Can you work these out from the model? Positions are in its coordinate system, mm. Face numbers are marked on the shaded views. A direction names the side the tool comes from. Coordinates: 2 decimals unless noted, no trailing zeros. Write each loop counter-clockwise with the first axis right and the second up, starting at its lowest first coordinate (ties: lowest second). Pieces come first, ordered by that corner, then holes. Notation, with made-up numbers: (25, 31) - (35, 31) arc R20 cw to (35, 51) - close; hole circle Ø6 at (25.25, 18.5). An arc over 180 degrees is marked (long way). Use one line per item in the form item = value. Start each with the question number.
(1) Thinking about a two-plate mould opening in X: for the marked faces 1, 2, 3 and 4, which applies, pulls with the +X half, pulls with the -X half, needs draft (parallel to the pull), parting line crosses it, or undercut?
(2) On a 3-axis mill with a long thin cutter (end or side, diameter ignored), from which of +Z, -Z, +X, -X, +Y, -Y can I reach the whole of each face in a straight line? I mean the marked faces 5, 6 and 7. Say none if no direction works.
(3) For pin 1 Ø2.5 at (x, y) = (-47.45, 55.69) entering from +Z; pin 2 Ø2 at (y, z) = (32.5, -28) entering from +X; pin 3 Ø17.5 at (y, z) = (37, -6) entering from +X; pin 4 Ø0.5 at (y, z) = (63.5, 3.5) entering from +X, each with a flat end and sliding along its axis, tell me the tip position at first contact or that it passes through.
(4) If we section it at A-A on z = -24.5: Please give me the cut outline in (x, y), then the cut area to 3 significant figures.
(5) If I drill on probe 1 along X at (y, z) = (-3, -12); probe 2 along X at (y, z) = (11.5, -16); probe 3 along Y at (x, z) = (54.5, -18), over which ranges is the centre line in solid material (lowest first)? Write a range as from..to.
Autodesk Fusion 360 part; units mm, degrees
sketch "Schizzo1" plane through (0, 0, 0) normal (0, 0, 1) x (1, 0, 0)
  line L0 (-31.0508, 65.6855) -> (44.1492, 65.6855)
  line L1 (44.1492, 65.6855) -> (44.1492, -9.3145)
  line L2 (44.1492, -9.3145) -> (-31.0508, -9.3145)
  line L3 (-31.0508, -9.3145) -> (-31.0508, 65.6855)
  line L4 (-31.0508, 28.1855) -> (44.1492, 28.1855) construction
  line L5 (6.5492, 65.6855) -> (6.5492, -9.3145) construction
  circle A0 centre (6.5492, 28.1855) radius 30.5
  line L6 (37.0492, -2.3145) -> (-23.9508, -2.3145) construction
  line L7 (-23.9508, -2.3145) -> (-23.9508, 58.6855) construction
  line L8 (-23.9508, 58.6855) -> (37.0492, 58.6855) construction
  line L9 (37.0492, 58.6855) -> (37.0492, -2.3145) construction
  line L10 (37.0492, -2.3145) -> (-23.9508, 58.6855) construction
  line L11 (-23.9508, -2.3145) -> (37.0492, 58.6855) construction
  circle A1 centre (-23.9508, 58.6855) radius 2.1
  circle A2 centre (37.0492, 58.6855) radius 2.1
  circle A3 centre (37.0492, -2.3145) radius 2.1
  circle A4 centre (-23.9508, -2.3145) radius 2.1
  line L12 (-71.9508, 58.6855) -> (-66.9508, 58.6855)
  line L13 (-66.9508, 58.6855) -> (-66.9508, -2.3145)
  line L14 (-66.9508, -2.3145) -> (-71.9508, -2.3145)
  line L15 (-71.9508, -2.3145) -> (-71.9508, 58.6855)
  line L16 (85.0492, 58.6855) -> (80.0492, 58.6855)
  line L17 (85.0492, -2.3145) -> (85.0492, 58.6855)
  line L18 (80.0492, 58.6855) -> (80.0492, -2.3145)
  line L19 (80.0492, -2.3145) -> (85.0492, -2.3145)
  circle A5 centre (-23.9508, 58.6855) radius 3.6
  circle A6 centre (37.0492, 58.6855) radius 3.6
  circle A7 centre (-23.9508, -2.3145) radius 3.6
  circle A8 centre (37.0492, -2.3145) radius 3.6
  line L20 (-31.0508, -9.3145) -> (-71.9508, -9.3145)
  line L21 (-71.9508, -9.3145) -> (-71.9508, -2.3145)
  line L22 (44.1492, -9.3145) -> (85.0492, -9.3145)
  line L23 (85.0492, -9.3145) -> (85.0492, -2.3145)
  line L24 (-66.9508, -2.3145) -> (-66.9508, -9.3145)
  line L25 (80.0492, -2.3145) -> (80.0492, -9.3145)
  line L26 (-66.9508, 58.6855) -> (-31.0508, 58.6855)
  line L27 (80.0492, 58.6855) -> (44.1492, 58.6855)
  line L28 (-66.9508, 58.6855) -> (-31.0508, 58.6855)
  line L29 (-31.0508, 58.6855) -> (-31.0508, 60.6855)
  line L30 (-31.0508, 60.6855) -> (-66.9508, 60.6855)
  line L31 (-66.9508, 60.6855) -> (-66.9508, 58.6855)
  line L32 (80.0492, 60.6855) -> (80.0492, 58.6855)
  line L33 (44.1492, 60.6855) -> (80.0492, 60.6855)
  line L34 (80.0492, 58.6855) -> (44.1492, 58.6855)
  line L35 (44.1492, -9.3145) -> (44.1492, 65.6855)
  line L36 (-36.0508, -9.3145) -> (-36.0508, 60.6855)
  line L37 (49.1492, -9.3145) -> (49.1492, 60.6855)
  line L38 (-71.9508, 58.6855) -> (-66.9508, 58.6855)
  line L39 (-66.9508, 58.6855) -> (-66.9508, 60.6855)
  line L40 (-66.9508, 60.6855) -> (-71.9508, 60.6855)
  line L41 (-71.9508, 60.6855) -> (-71.9508, 58.6855)
  line L42 (85.0492, 60.6855) -> (85.0492, 58.6855)
  line L43 (80.0492, 60.6855) -> (85.0492, 60.6855)
  point P0 (6.5492, 28.1855)
  point P1 (-23.9508, -2.3145)
  dimension "d1" = 75.2
  dimension "d2" = 75
  dimension "d3" = 61
  dimension "d4" = 61
  dimension "d5" = 61
  dimension "d6" = 4.2
  dimension "d13" = 5
  dimension "d22" = 7.2
  dimension "d70" = 157
  dimension "d82" = 147
  dimension "d102" = 2
  dimension "d109" = 5
extrude "Estrusione1" add sketch "Schizzo1" along normal blind 6 contours L0 L1 L2 L3 L29 L35 | L3 L26 L28 L29 L30 L36 | L1 L27 L33 L34 L35 L37 | L3 L20 L26 L28 L36 | L1 L22 L27 L34 L35 L37 | A5 | A6 | A7 | A8
fillet "Raccordo22" radius 2 1 edges at (-21.8868, 39.2148, 6)
extrude "Estrusione14" add sketch "Schizzo1" against normal blind 20 contours L3 L26 L28 L29 L30 L36 | L1 L27 L33 L34 L35 L37 | L3 L20 L26 L28 L36 | L1 L22 L27 L34 L35 L37
fillet "Raccordo20" radius 2 2 edges at (-31.0508, 25.6855, 0) (44.1492, 25.6855, 0)
fillet "Raccordo17" radius 2 2 edges at (-31.0508, 65.6855, 3) (44.1492, 65.6855, 3)
fillet "Raccordo21" radius 2 2 edges at (44.1492, 60.6855, 3) (-31.0508, 60.6855, 3)
extrude "Estrusione15" add sketch "Schizzo1" along normal blind 6 from surface at -20 contours L3 L20 L26 L28 L36 | L26 L28 L30 L31 L36 L39 | L1 L22 L27 L34 L35 L37 | L27 L32 L33 L34 L37 | L13 L20 L24 L26 L28 L36 | L12 L31 L38 L39 L40 L41 | L18 L22 L25 L27 L34 L37 | L16 L32 L42 L43 | L12 L13 L14 L15 L38 | L16 L17 L18 L19 | L14 L20 L21 L24 | L19 L22 L23 L25
fillet "Raccordo14" radius 2 2 edges at (49.1492, 25.6855, -14) (-36.0508, 25.6855, -14)
fillet "Raccordo18" radius 2 2 edges at (44.1492, 25.6855, -20) (-31.0508, 25.6855, -20)
extrude "Estrusione2" add sketch "Schizzo1" against normal blind 20 from surface at -15 contours L12 L31 L38 L39 L40 L41 | L16 L32 L42 L43 | L12 L13 L14 L15 L38 | L16 L17 L18 L19 | L14 L20 L21 L24 | L19 L22 L23 L25
fillet "Raccordo23" radius 2 2 edges at (-71.9508, 25.6855, -14) (85.0492, 25.6855, -14)
fillet "Raccordo24" radius 2 2 edges at (-66.9508, 25.6855, -20) (80.0492, 25.6855, -20)
sketch "Schizzo2" plane through (-71.9508, 0, 0) normal (-1, 0, 0) x (0, -1, 0)
  line L0 (-60.6855, -35) -> (9.3145, -35)
  circle A0 centre (-28.1855, -30) radius 2.9
  circle A1 centre (-28.1855, -30) radius 3.5
  line L1 (9.3145, -35) -> (9.3145, -16)
  circle A2 centre (0.8145, -30) radius 1.9
  line L2 (-58.6855, -15) -> (9.3145, -15) construction
  line L3 (9.3145, -15) -> (9.3145, -35) construction
  line L4 (9.3145, -35) -> (-58.6855, -35) construction
  line L5 (-58.6855, -35) -> (-58.6855, -15) construction
  line L6 (-58.6855, -30) -> (9.3145, -30) construction
  line L7 (9.3145, -16) -> (-60.6855, -16)
  line L8 (-60.6855, -16) -> (-60.6855, -35)
  dimension "d27" = 5.8
  dimension "d28" = 7
  dimension "d56" = 3.8
  dimension "d94" = 5
  dimension "d95" = 30.5
  dimension "d96" = 29
extrude "Estrusione4" add sketch "Schizzo2" along normal blind 7 contours A0
extrude "Estrusione5" add sketch "Schizzo2" against normal blind 2 from surface at 7 contours A1
fillet "Raccordo4" radius 0.5 1 edges at (-71.9508, 30.8893, -28.9513)
extrude "Estrusione10" cut sketch "Schizzo2" against normal blind 3.5 contours A2
sketch "Schizzo3" plane through (85.0492, 0, 0) normal (1, 0, 0) x (0, 1, 0)
  line L0 (-9.3145, -35) -> (60.6855, -35)
  circle A0 centre (28.1855, -30) radius 2.9
  circle A1 centre (28.1855, -30) radius 3.5
  circle A2 centre (-0.8145, -30) radius 1.9
  line L1 (-9.3145, -16) -> (-9.3145, -35)
  line L2 (58.6855, -35) -> (-9.3145, -35) construction
  line L3 (-9.3145, -35) -> (-9.3145, -15) construction
  line L4 (-9.3145, -15) -> (58.6855, -15) construction
  line L5 (58.6855, -15) -> (58.6855, -35) construction
  line L6 (-9.3145, -30) -> (58.6855, -30) construction
  line L7 (60.6855, -16) -> (-9.3145, -16)
  line L8 (60.6855, -35) -> (60.6855, -16)
  dimension "d36" = 5.8
  dimension "d37" = 7
  dimension "d49" = 3.8
  dimension "d97" = 5
  dimension "d98" = 29
  dimension "d99" = 30.5
extrude "Estrusione6" add sketch "Schizzo3" along normal blind 7 contours A0
extrude "Estrusione7" add sketch "Schizzo3" against normal blind 2 from surface at 7 contours A1
fillet "Raccordo5" radius 0.5 1 edges at (85.0492, 25.4818, -28.9513)
extrude "Estrusione11" cut sketch "Schizzo3" against normal blind 3.5 contours A2
sketch "Schizzo4" plane through (0, 0, 6) normal (0, 0, 1) x (-1, 0, 0)
  line L0 (36.0508, 9.3145) -> (-49.1492, 9.3145)
  line L1 (-42.1492, -65.6855) -> (29.0508, -65.6855)
  circle A0 centre (23.9508, 2.3145) radius 2.1
  circle A1 centre (-37.0492, -58.6855) radius 2.1
  circle A2 centre (23.9508, -58.6855) radius 2.1
  circle A3 centre (-37.0492, 2.3145) radius 2.1
  line L2 (65.9508, -65.6855) -> (-79.0492, -65.6855) construction
  line L3 (-79.0492, -65.6855) -> (-79.0492, 9.3145) construction
  line L4 (-79.0492, 9.3145) -> (65.9508, 9.3145) construction
  line L5 (65.9508, 9.3145) -> (65.9508, -65.6855) construction
  line L6 (-6.5492, -65.6855) -> (-6.5492, 9.3145) construction
  line L7 (-6.5492, -28.1855) -> (65.9508, -28.1855) construction
  line L8 (-6.5492, -28.1855) -> (-79.0492, -28.1855) construction
  line L9 (65.9508, -55.6855) -> (-79.0492, -55.6855) construction
  line L10 (65.9508, -0.6855) -> (-79.0492, -0.6855) construction
  circle A4 centre (47.4508, -55.6855) radius 2.25
  circle A5 centre (47.4508, -55.6855) radius 3.75
  circle A6 centre (51.4508, -0.6855) radius 2.25
  circle A7 centre (51.4508, -0.6855) radius 3.75
  circle A8 centre (-60.5492, -55.6855) radius 2.25
  circle A9 centre (-60.5492, -55.6855) radius 3.75
  circle A10 centre (-64.5492, -0.6855) radius 3.75
  circle A11 centre (-64.5492, -0.6855) radius 2.25
  line L11 (-44.1492, -62.6855) -> (-44.1492, -63.6855)
  line L12 (31.0508, -63.6855) -> (31.0508, -62.6855)
  line L13 (-49.1492, 9.3145) -> (-49.1492, -60.6855)
  line L14 (36.0508, -60.6855) -> (36.0508, 9.3145)
  arc A12 (-44.1492, -63.6855) -> (-42.1492, -65.6855) centre (-42.1492, -63.6855) ccw
  arc A13 (29.0508, -65.6855) -> (31.0508, -63.6855) centre (29.0508, -63.6855) ccw
  circle A14 centre (-6.5492, -28.1855) radius 32.5
  arc A15 (33.0508, -60.6855) -> (31.0508, -62.6855) centre (33.0508, -62.6855) ccw
  line L15 (33.0508, -60.6855) -> (36.0508, -60.6855)
  line L16 (-49.1492, -60.6855) -> (-46.1492, -60.6855)
  arc A16 (-44.1492, -62.6855) -> (-46.1492, -60.6855) centre (-46.1492, -62.6855) ccw
  point P0 (47.4508, -55.6855)
  point P1 (51.4508, -0.6855)
  point P2 (-60.5492, -55.6855)
  point P3 (-64.5492, -0.6855)
  dimension "d79" = 55
  dimension "d80" = 108
  dimension "d81" = 116
  dimension "d83" = 4.5
  dimension "d84" = 7.5
  dimension "d85" = 4.5
  dimension "d86" = 7.5
extrude "Estrusione12" cut sketch "Schizzo4" against normal blind 6 from surface at -20 contours A4 | A6 | A8 | A11
equation "d1 = 75 mm + 0.2 mm"
equation "d85 = d83"
equation "d86 = d84"
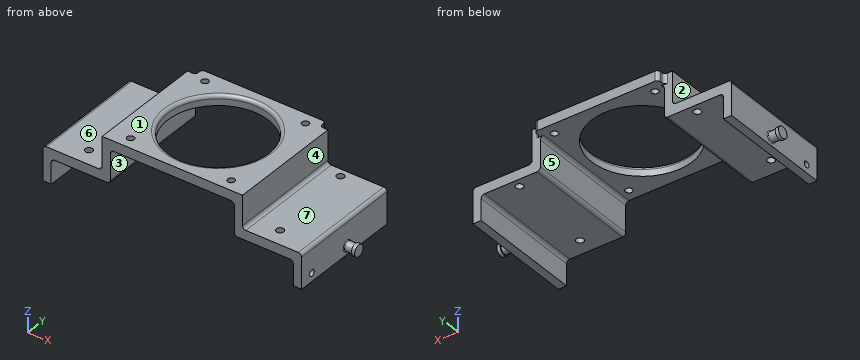
Reported:
q1.face_1 = needs draft
q1.face_2 = pulls with the -X half
q1.face_3 = undercut
q1.face_4 = pulls with the +X half
q2.face_5 = -Z, +Y, -Y
q2.face_6 = +Z, -X, +Y, -Y
q2.face_7 = +Z, +X, +Y, -Y
q3.pin_1 = through
q3.pin_2 = 85.05
q3.pin_3 = 84.61
q3.pin_4 = 44.15
q4.outline = (-71.95, -9.31) - (-66.95, -9.31) - (-66.95, 60.69) - (-71.95, 60.69) - close; (80.05, -9.31) - (85.05, -9.31) - (85.05, 60.69) - (80.05, 60.69) - close
q4.area = 700 mm2
q5.probe_1 = -36.05..-31.05, 44.15..49.15
q5.probe_2 = -71.95..-31.05, 44.15..85.05
q5.probe_3 = -9.31..60.69
